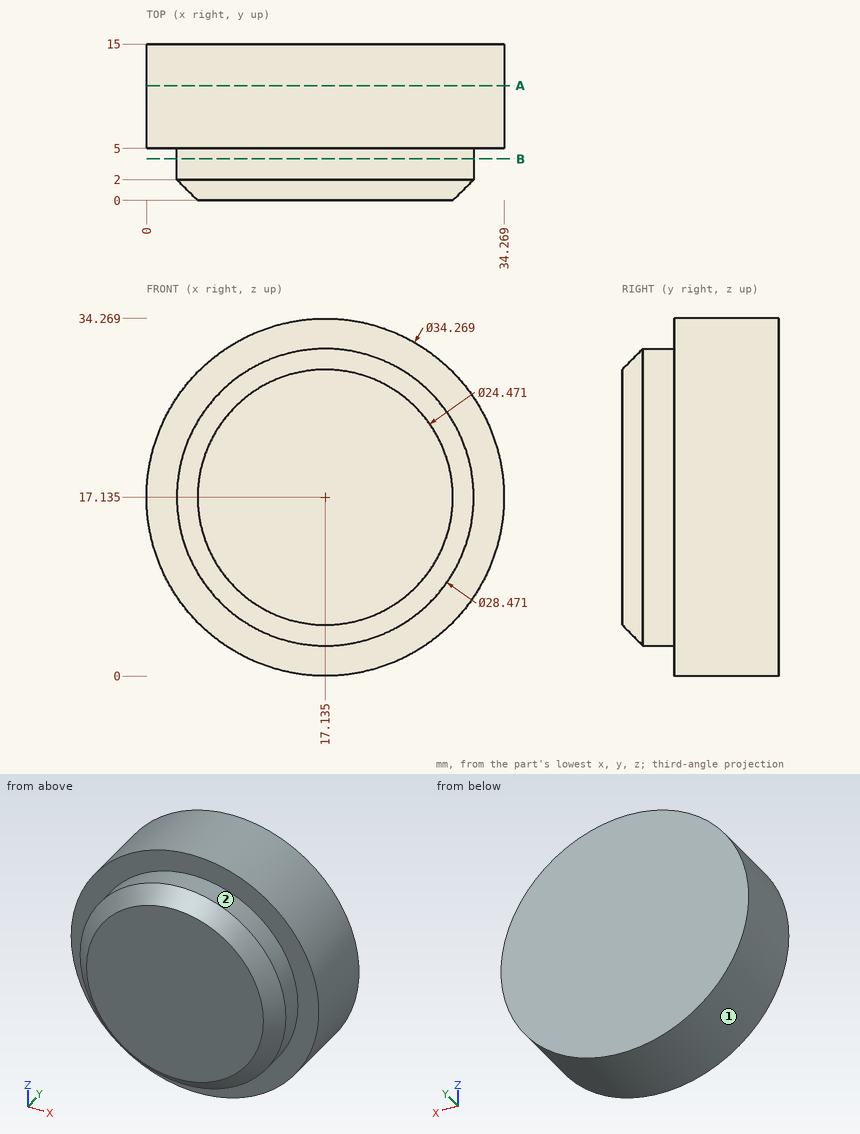
Geometry check sheet. Reference: drawing and pictorial views, mm from the part's lowest x, y, z. A direction names the side the tool comes from. Give positions to 0.01 mm unless a question says otherwise; leave off trailing zeros. Order: outer loops, then holes, each group sorted by start corner. A loop starts at its lowest first (then second) coordinate and runs counter-clockwise, first axis right, second up. Notation, with made-up numbers: M 56.25,-1 L 60.25,-1 A34 ccw 60.25,36 Z; hole C 77.5,5.5 d11. An arc over 180 degrees is marked long. Answer as a JSON object with one key per item and string values. Group by question number.
1) Depth check by flat-ended pin: pin 1 Ø8 at (y, z) = (11.5, 8.5) entering from +X; pin 2 Ø1.5 at (x, z) = (4, 20) entering from -Y; pin 3 Ø5 at (x, y) = (29, 2) entering from -Z (1 decimal). Enter the tip coordinate at first touch or a pass-through.
2) Cross-section at A-A (y = 11). Enter the section's corners in (x, z) (1 decimal), then the cut area to 3 significant figures.
3) Access from +Z, -Z, +X, -X, +Y, -Y to the whole of each face (thin tool, end or side, straight path). Record for the marked faces 1 and 2.
4) Cross-section at B-B (y = 4). Enter the section's corners in (x, z) (1 decimal).
5) Scan lines: line 1 along Z through (x, y) = (17, 8.5); line 2 along Y through (x, z) = (2, 12.5); line 3 along X through (y, z) = (7.25, 23) (1 decimal). Record each from-to range of solid material in increasing order. Write a range as [from, to].
Result sheet:
{
 "1": {"pin 1": "stops at x = 33.63", "pin 2": "stops at y = 0.46", "pin 3": "stops at z = 6.4"},
 "2": {"outline": "C 17.1,17.1 d34.3", "area": "922 mm2"},
 "3": {"face 1": "+Y, -Y", "face 2": "-Y"},
 "4": {"outline": "C 17.1,17.1 d28.5"},
 "5": {"line 1": "z = [0, 34.27]", "line 2": "y = [5, 15]", "line 3": "x = [1, 33.2]"}
}
